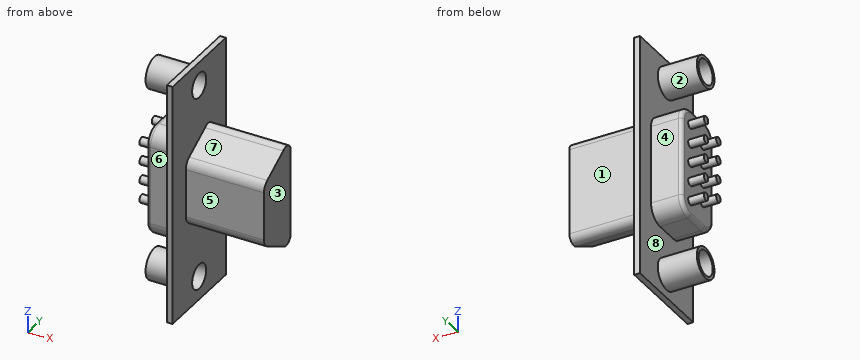
```python
from build123d import *

# Parameters (mm, degrees)
SKETCH1_W                    = 31
SKETCH1_H                    = 12
BASE_FLANGE1_DEPTH           = 0.7366
EXTRUDE_THIN3_DEPTH          = 10
SKETCH8_W                    = 14
SKETCH8_H                    = 7
BOSS_EXTRUDE1_DEPTH          = 4
FILLET2_R                    = 2
FILLET3_R                    = 0.5
SKETCH9_R                    = 0.498553058
BOSS_EXTRUDE2_DEPTH          = 2
SKETCH10_R                   = 0.49857
BOSS_EXTRUDE3_DEPTH          = 2
SKETCH11_R                   = 1.984375
BOSS_EXTRUDE4_DEPTH          = 5
F_1_8_0_125_DIAMETER_HOLE1_D = 3.175


# Sheet-metal steps are written as plain solids
with BuildPart() as part:
    # Sketch1 → Base-Flange1 (new body)
    with BuildSketch(Plane(origin=(0, 0, 0), x_dir=(0, 0, -1), z_dir=(1, 0, 0))):
        Rectangle(SKETCH1_W, SKETCH1_H)
    extrude(amount=-BASE_FLANGE1_DEPTH)

    # Sketch6 → Extrude-Thin3 (add)
    with BuildSketch(Plane(origin=(0, 0, 0), x_dir=(0, 0, -1), z_dir=(1, 0, 0))):
        with BuildLine():
            Line((0, 3), (5.5, 3))
            ThreePointArc((5.5, 3), (6.414535338, 2.404506015), (6.23987009, 1.327250232))
            Line((6.23987009, 1.327250232), (4.317359578, -2.26115081))
            ThreePointArc((4.317359578, -2.26115081), (3.802471809, -2.801168417), (3.083309495, -3))
            Line((3.083309495, -3), (0, -3))
            Line((0, -3), (0, -0.001))
            Line((0, -0.001), (2.125957868, -0.001))
            Line((2.125957868, -0.001), (2.127029382, 0.001))
            Line((2.127029382, 0.001), (0, 0.001))
            Line((0, 0.001), (0, 3))
        make_face()
    extrude_thin3 = extrude(amount=EXTRUDE_THIN3_DEPTH)

    # Mirror1: Extrude-Thin3 across plane
    add(extrude_thin3.mirror(Plane.XY))

    # Sketch8 → Boss-Extrude1 (add)
    with BuildSketch(Plane.ZY.offset(0.7366)):
        Rectangle(SKETCH8_W, SKETCH8_H)
    extrude(amount=BOSS_EXTRUDE1_DEPTH)

    # Fillet2
    fillet2_edges = [part.edges().sort_by_distance(p)[0] for p in [
        (-2.7366, -3.5, 7),
        (-2.7366, 3.5, 7),
        (-2.7366, 3.5, -7),
        (-2.7366, -3.5, -7),
    ]]
    fillet(fillet2_edges, radius=FILLET2_R)

    # Fillet3
    fillet3_edges = [part.edges().sort_by_distance(p)[0] for p in [
        (-4.7366, 0, 7),
        (-4.7366, -3.5, 0),
        (-4.7366, 3.5, 0),
        (-4.7366, 0, -7),
        (-4.7366, 2.914213562, -6.414213562),
        (-4.7366, -2.914213562, -6.414213562),
        (-4.7366, 2.914213562, 6.414213562),
        (-4.7366, -2.914213562, 6.414213562),
    ]]
    fillet(fillet3_edges, radius=FILLET3_R)

    # Sketch9 → Boss-Extrude2 (add)
    with BuildSketch(Plane.ZY.offset(4.7366)):
        with Locations(Location((-5, 1.673069628, 0), (0, 0, 180))):
            Circle(SKETCH9_R)
        with Locations(Location((-2.5, 1.673069628, 0), (0, 0, 180))):
            Circle(SKETCH9_R)
        with Locations(Location((0, 1.673069628, 0), (0, 0, 180))):
            Circle(SKETCH9_R)
        with Locations(Location((2.5, 1.673069628, 0), (0, 0, 180))):
            Circle(SKETCH9_R)
        with Locations(Location((5, 1.673069628, 0), (0, 0, 180))):
            Circle(SKETCH9_R)
    extrude(amount=BOSS_EXTRUDE2_DEPTH)

    # Sketch10 → Boss-Extrude3 (add)
    with BuildSketch(Plane.ZY.offset(4.7366)):
        with Locations(Location((-3.75, -1.115638979, 0), (0, 0, 180))):
            Circle(SKETCH10_R)
        with Locations(Location((-1.25, -1.115638979, 0), (0, 0, 180))):
            Circle(SKETCH10_R)
        with Locations(Location((1.25, -1.115638979, 0), (0, 0, 180))):
            Circle(SKETCH10_R)
        with Locations(Location((3.75, -1.115638979, 0), (0, 0, 180))):
            Circle(SKETCH10_R)
    extrude(amount=BOSS_EXTRUDE3_DEPTH)

    # Sketch11 → Boss-Extrude4 (add)
    with BuildSketch(Plane.ZY.offset(0.7366)):
        with Locations((-12.5, 0)):
            Circle(SKETCH11_R)
    boss_extrude4 = extrude(amount=BOSS_EXTRUDE4_DEPTH)

    # Mirror2: Boss-Extrude4 across plane
    add(boss_extrude4.mirror(Plane.XY))

    # 1/8 (0.125) Diameter Hole1 (through all)
    with Locations(Plane.ZY.offset(5.7366)):
        with Locations((-12.5, 0)):
            f_1_8_0_125_diameter_hole1 = Hole(F_1_8_0_125_DIAMETER_HOLE1_D / 2)

    # Mirror3: 1/8 (0.125) Diameter Hole1 across plane
    add(f_1_8_0_125_diameter_hole1.mirror(Plane.XY), mode=Mode.SUBTRACT)


solid = part.part
```
Part model, mm, in its own coordinate system. Face numbers are marked on the shaded views. A direction names the side the tool comes from. Round coordinates to 2 decimals unless told otherwise and drop trailing zeros. Order: outer loops, then holes, each group sorted by start corner. A loop starts at its lowest first (then second) coordinate and runs counter-clockwise, first axis right, second up. Notation, with made-up numbers: M -12.75,-7.75 L 46.25,-7.75 A15 cw 46.25,9.25 Z; hole C 8.5,27 d6. An arc over 180 degrees is marked long. Answer in a Markdown table with one row per item. Add a question column.
Q1. Cut at A-A on z = -12. Give the cut face in (x, y).
Q2. Cut at C-C on y = 0.5. Give the number of separate pieces and of enclosed holes in the cut face, and give its area (3 significant figures).
Q3. Cut at D-D on z = 2.5. Give the cut face in (x, y), and give its area (3 significant figures).
Q4. Mould opens along Z. For the marked faces 6, 7 and 8 say: +Z half, -Z half, draft (parallel to the pull), parting line (faces both ways), or undercut.
Q5. 3-axis set-ups, long thin cutter, end or side, ignore diameter. For the marked faces 1, 2, 3, 4 and 5: which of +Z, -Z, +X, -X, +Y, -Y reach the whole face in a straight line?
Q6. Pin check, flat tips, straight feed: pin 1 (1 mm diameter, centred on x = 7, z = 2, fed in from +Y); pin 2 (1.3 mm diameter, centred on x = 3.5, z = -0.5, fed in from -Y); pin 3 (4.5 mm diameter, centred on y = -0.5, z = 13, fed in from -X). Stop position of each tip, or through.
Q7. Wall check: L1, parallel to Y at x = -3.5, z = -12.5; L2, parallel to Y at x = -3.25, z = 3; L3, parallel to X at y = 0, z = 3. Give the ranges that are in metal, low to high. Write a range as from..to.
Established:
| question | item | result |
|---|---|---|
| 1 | outline | M -5.74,-1.92 L -0.74,-1.92 L -0.74,-6 L 0,-6 L 0,-1.51 L -5.74,-1.51 Z; M -5.74,1.51 L 0,1.51 L 0,6 L -0.74,6 L -0.74,1.92 L -5.74,1.92 Z |
| 2 | separate pieces | 3 |
| 2 | enclosed holes | 0 |
| 2 | area | 198 mm2 |
| 3 | outline | M -6.74,1.17 L -4.74,1.17 L -4.74,-3 A0.5 ccw -4.24,-3.5 L -0.74,-3.5 L -0.74,-6 L 0,-6 L 0,-3 L 10,-3 L 10,3 L 0,3 L 0,6 L -0.74,6 L -0.74,3.5 L -4.24,3.5 A0.5 ccw -4.74,3 L -4.74,2.17 L -6.74,2.17 Z |
| 3 | area | 98.7 mm2 |
| 4 | face 6 | draft |
| 4 | face 7 | +Z half |
| 4 | face 8 | undercut |
| 5 | face 1 | +Z, -Z, +X, +Y |
| 5 | face 2 | -X |
| 5 | face 3 | +Z, -Z, +X, +Y, -Y |
| 5 | face 4 | +Z, -Z, -X, +Y |
| 5 | face 5 | +Z, -Z, +X, -Y |
| 6 | pin 1 | stops at y = 3 |
| 6 | pin 2 | stops at y = -3 |
| 6 | pin 3 | stops at x = -5.74 |
| 7 | L1 | y = -1.98..-1.59, 1.59..1.98 |
| 7 | L2 | y = -3.5..3.5 |
| 7 | L3 | x = -4.74..10 |
